from build123d import *

# Parameters (mm, degrees)
BODY_DEPTH          = 18.4404
SKETCH3_R           = 5.1435
SKETCH3_R_2         = 0.7493
BOSS_EXTRUDE2_DEPTH = 1.524
SKETCH4_R           = 4.7625
MOUNT_LUG_DEPTH     = 6.4008
SKETCH5_R           = 3.175
SHAFT_DEPTH         = 12.7
FILLET1_R           = 0.762
SKETCH6_W           = 0.8128
SKETCH6_H           = 1.6256
ADJ_SLOT_DEPTH      = 12.2395
ADJ_SLOT_DEPTH_BACK = 12.2395
CHAMFER1_SIZE       = 0.762


with BuildPart() as part:
    # Sketch1 → Body (new body)
    with BuildSketch(Plane(origin=(0, 0, 0), x_dir=(1, 0, 0), z_dir=(0, 1, 0))):
        with BuildLine():
            Line((3.429, 12.7), (-3.429, 12.7))
            Line((-3.429, 12.7), (-3.429, 10.703659152))
            ThreePointArc((-3.429, 10.703659152), (0, -11.2395), (3.429, 10.703659152))
            Line((3.429, 10.703659152), (3.429, 12.7))
        make_face()
    extrude(amount=BODY_DEPTH)

    # Sketch3 → Boss-Extrude2 (add)
    with BuildSketch(Plane(origin=(0, 18.4404, 0), x_dir=(1, 0, 0), z_dir=(0, 1, 0))):
        Circle(SKETCH3_R)
        with Locations((0, 7.366)):
            Circle(SKETCH3_R_2)
    extrude(amount=BOSS_EXTRUDE2_DEPTH)

    # Sketch4 → Mount Lug (add)
    with BuildSketch(Plane(origin=(0, 19.9644, 0), x_dir=(1, 0, 0), z_dir=(0, 1, 0))):
        Circle(SKETCH4_R)
    extrude(amount=MOUNT_LUG_DEPTH)

    # Sketch5 → Shaft (add)
    with BuildSketch(Plane(origin=(0, 26.3652, 0), x_dir=(1, 0, 0), z_dir=(0, 1, 0))):
        Circle(SKETCH5_R)
    extrude(amount=SHAFT_DEPTH)

    # Fillet1
    fillet1_edges = [part.edges().sort_by_distance(p)[0] for p in [
        (-3.175, 39.0652, 0),
    ]]
    fillet(fillet1_edges, radius=FILLET1_R)

    # Sketch6 → Adj. slot (cut, two sides)
    with BuildSketch(Plane(origin=(0, 0, 0), x_dir=(0, 0, -1), z_dir=(1, 0, 0))) as adj_slot_sk:
        with Locations((0, 39.0652)):
            Rectangle(SKETCH6_W, SKETCH6_H)
    extrude(amount=ADJ_SLOT_DEPTH, mode=Mode.SUBTRACT)
    extrude(adj_slot_sk.sketch, amount=-ADJ_SLOT_DEPTH_BACK, mode=Mode.SUBTRACT)

    # Chamfer1
    chamfer1_edges = [part.edges().sort_by_distance(p)[0] for p in [
        (0, 18.4404, 11.2395),
        (0, 0, 11.2395),
    ]]
    chamfer(chamfer1_edges, length=CHAMFER1_SIZE)


solid = part.part
For this review, take the finished solid that the model builds, in its own axes (mm). A direction names the side the tool comes from. Coordinates: 2 decimals unless noted, no trailing zeros. Order: outer loops, then holes, each group sorted by start corner. A loop starts at its lowest first (then second) coordinate and runs counter-clockwise, first axis right, second up. Notation, with made-up numbers: (-28.75, 36.25) - (-16.75, 36.25) arc R18 ccw to (-16.75, 51.25) - close; hole circle Ø11 at (-33.75, 59.5). An arc over 180 degrees is marked (long way). Answer as CSV lines item,"result". Start each with the question number.
1) Machinability: for faces 4 (the cylindrical face through (-0.67, 19.19, -5.1)), 5 (the flat face through (0, 19.964, -7)), 6 (the flat face through (0, 9, -12.7)), 7 (the flat face through (0, 38.7, 0.406)), 8 (the flat face through (0, 39.065, 1)), which of the approach directions +Z, -Z, +X, -X, +Y, -Y give a long, thin tool a straight path to every point of the face, cutting with its end or side? Answer none if there is none.
2) Insertion check: P1, Ø1.5, axis at y = 23.5, z = 2.5, coming from the -X side; P2, Ø3, axis at y = 34, z = 1.5, coming from the -X side (3 decimals); P3, Ø3, axis at y = 12, z = -11, coming from the +X side. Each pin has a flat end and moves straight along its axis. Give the tip position at first contact, or say it passes through.
3) Add section C-C (y = 31). State the section outline as (x, z) points (3 decimals), then the cut area to 3 significant figures.
4) To check wall thickness, follow line 1 along Y through (x, z) = (-8, 3.5); line 2 along Z through (x, y) = (-0.25, 12.5); line 3 along Y through (x, z) = (-3.25, -0.25). State the ranges of each line that lie inside material, in increasing order. Write a range as [from, to].
5) Draft analysis for pull direction Z (two halves, no side actions). For faces 1 (the conical face through (-0.42, 0.12, 10.59)), 2 (the flat face through (0, 39.065, -1)), 3 (the flat face through (0, 38.252, 0)), state which applies: +Z half, -Z half, draft (parallel to the pull), parting line (faces both ways), or undercut.
6) Add section B-B (y = 17). State the section outline as (x, z) points.
Result:
1,face 4,"+Y"
1,face 5,"-Z, +X, -X, +Y"
1,face 6,"-Z, +X, -X, +Y, -Y"
1,face 7,"+X, -X, +Y"
1,face 8,"+Z, -Z, +X, -X, +Y"
2,P1,"x = -4.43"
2,P2,"x = -3.175"
2,P3,"x = 6.01"
3,outline,"circle Ø6.35 at (0, 0)"
3,area,"31.7 mm^2"
4,line 1,"[0, 18.44]"
4,line 2,"[-12.7, 11.24]"
4,line 3,"[0, 26.37]"
5,face 1,"parting line"
5,face 2,"draft"
5,face 3,"undercut"
6,outline,"(-3.43, -12.7) - (3.43, -12.7) - (3.43, -10.7) arc R11.24 ccw (long way) to (-3.43, -10.7) - close"
